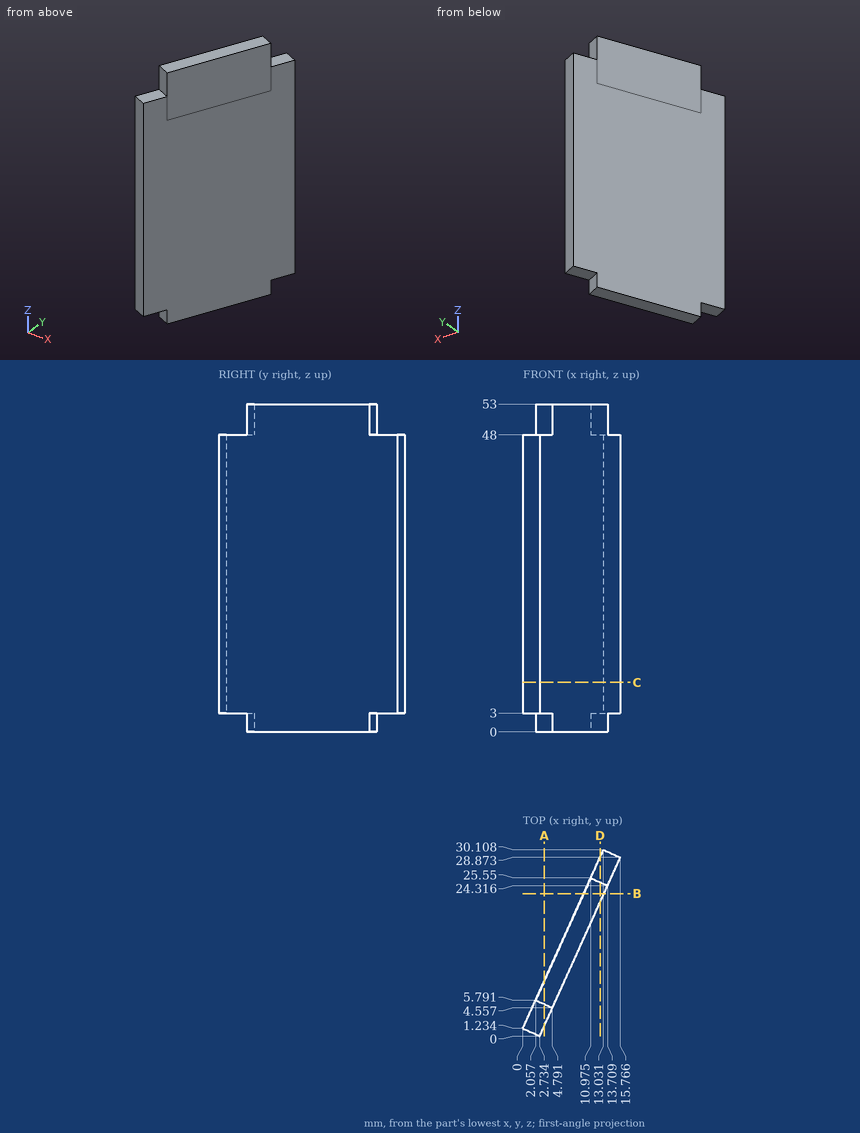
Check sheet for the drawn part. Datum: minimum x, y, z corner. Units: mm. Round coordinates to 2 decimals unless told otherwise and drop trailing zeros. Order: outer loops, then holes, each group sorted by start corner. A loop starts at its lowest first (then second) coordinate and runs counter-clockwise, first axis right, second up. Notation, with made-up numbers: (42.25, 79.5) -> (49.25, 79.5) arc R24 ccw to (49.25, 105.5) -> close; hole circle Ø1 at (60.25, 45). An arc over 180 degrees is marked (long way). Return JSON: item names as keys, results as strings. Group by question number.
Q1. Section check C-C, the plane z = 8. Record the boundary of the cut face in (x, y) (1 decimal).
Q2. Section check B-B, the plane y = 23. Record the boundary of the cut face in (x, z) (1 decimal).
Q3. Material ranges on probe 1 along Y at (x, z) = (11, 15.5) (1 decimal); probe 2 along Z at (x, y) = (3.25, 4.5); probe 3 along X at (y, z) = (21.5, 5) (1 decimal), recorded low to high. Write a range as from..to.
Q4. Section check D-D, the plane x = 12.5. Record the boundary of the cut face in (y, z).
Q5. Gauge pin test, flat ends, axial feed: pin 1 (2.5 mm diameter, centred on x = 14, y = 26.5, fed in from -Z); pin 2 (3 mm diameter, centred on x = 8, z = 15.5, fed in from +Y) (1 decimal); pin 3 (5 mm diameter, centred on x = 6, z = 8.5, fed in from -Y) (1 decimal). Record the tip position at first contact, or that the pin passes through.
Q6. Section check A-A, the plane x = 3.5. Record the boundary of the cut face in (y, z).
Numbers:
{
 "1": {"outline": "(0, 1.2) -> (2.7, 0) -> (15.8, 28.9) -> (13, 30.1) -> close"},
 "2": {"outline": "(9.8, 0) -> (13.1, 0) -> (13.1, 53) -> (9.8, 53) -> close"},
 "3": {"probe 1": "18.3..25.6", "probe 2": "3..48", "probe 3": "9.1..12.4"},
 "4": {"outline": "(21.64, 0) -> (24.86, 0) -> (24.86, 3) -> (28.93, 3) -> (28.93, 48) -> (24.86, 48) -> (24.86, 53) -> (21.64, 53) -> close"},
 "5": {"pin 1": "z = 3", "pin 2": "y = 22.3", "pin 3": "y = 1.7"},
 "6": {"outline": "(1.7, 3) -> (5.14, 3) -> (5.14, 0) -> (8.99, 0) -> (8.99, 53) -> (5.14, 53) -> (5.14, 48) -> (1.7, 48) -> close"}
}
